Part model, mm, in its own coordinate system. Face numbers are marked on the shaded views. A direction names the side the tool comes from. Give positions to 0.01 mm unless a question says otherwise; leave off trailing zeros. Order: outer loops, then holes, each group sorted by start corner. A loop starts at its lowest first (then second) coordinate and runs counter-clockwise, first axis right, second up. Notation, with made-up numbers: (-5.5, -34.75) -> (8.5, -34.75) arc R30 ccw to (8.5, 3.25) -> close; hole circle Ø8 at (17, 66.25). An arc over 180 degrees is marked (long way). Write item = value, one per line. Start each with the question number.
(1) Saw through at A-A, the plane y = 0. List the corners of the cut face in (x, z), then the cut area to 3 significant figures.
(2) Which spindle directions (+Z, -Z, +X, -X, +Y, -Y) get a long thin tool onto all of the face, cutting with end or side? Do the marked faces 4 and 5. Say none if no direction does.
(3) Two-plate mould, pull along X, no slides. Class the marked faces 1, 2 and 3: pulls with the +X half, pulls with the -X half, needs draft (parallel to the pull), parting line crosses it, or undercut.
(4) Saw through at D-D, the plane z = -104. List the corners of the cut face in (x, y).
(5) Saw through at C-C, the plane z = -10. List the corners of the cut face in (x, y).
(6) Flat gauge pins, fed straight in: pin 1 (6 mm diameter, centred on x = 23.5, z = -104, fed in from -Y); pin 2 (12 mm diameter, centred on y = -24.5, z = -107, fed in from -X); pin 3 (8 mm diameter, centred on y = -6, z = -66.5, fed in from +X); pin 4 (12 mm diameter, centred on x = -2.5, y = 14, fed in from +Z). Where does each tip first touch, or does it go through?
(7) Probe line 1 along Y through (x, z) = (0, -35); line 2 along Y through (x, z) = (0, -107); line 3 along Z through (x, y) = (-27, 24). List the from-to ranges inside material, lowest first. Write a range as from..to.
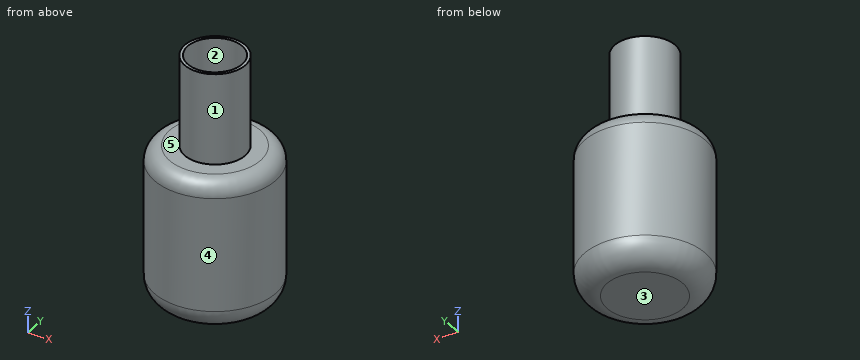
Autodesk Fusion 360 part; units mm, degrees
sketch "Sketch1" plane through (0, 0, 0) normal (0, 1, 0) x (1, 0, 0)
  line L0 (0, 0) -> (20, 0)
  line L1 (20, 0) -> (20, 60)
  line L2 (20, 60) -> (40, 60)
  line L3 (40, 60) -> (40, 160)
  line L4 (40, 160) -> (0, 160)
  line L5 (0, 160) -> (0, 0)
  dimension "d8" = 100
  dimension "d9" = 160
  dimension "d10" = 20
revolve "Revolve1" add sketch "Sketch1" angle 360 about axis through (0, 0, -160) along (0, 0, 1)
fillet "Fillet1" radius 10 1 edges at (-37.2931, -14.4646, -60)
fillet "Fillet2" radius 15 1 edges at (-37.2931, -14.4646, -160)
shell "Shell1" thickness 2 removed faces 1 at (3.8604, -3.2472, 0)
equation "overalheight = 160 mm"
equation "neckheight = 100 mm"
equation "fillet1 = 15 mm"
equation "fillet2 = 10 mm"
equation "fillet3 = 5 mm"
equation "diameter = 20 mm"
equation "wallthickness = 2 mm"
equation "d8 = neckheight"
equation "d9 = overalheight"
equation "d10 = diameter"
equation "d12 = fillet2"
equation "d13 = fillet1"
equation "d14 = wallthickness"
Results list:
q1.outline = (-40, -145) arc R15 ccw to (-25, -160) -> (25, -160) arc R15 ccw to (40, -145) -> (40, -70) arc R10 ccw to (30, -60) -> (20, -60) -> (20, 0) -> (18, 0) -> (18, -62) -> (30, -62) arc R8 cw to (38, -70) -> (38, -145) arc R13 cw to (25, -158) -> (-25, -158) arc R13 cw to (-38, -145) -> (-38, -70) arc R8 cw to (-30, -62) -> (-18, -62) -> (-18, 0) -> (-20, 0) -> (-20, -60) -> (-30, -60) arc R10 ccw to (-40, -70) -> close
q1.area = 833 mm^2
q2.face_4 = +Z, -Z
q2.face_5 = +Z
q3.face_1 = parting line crosses it
q3.face_2 = undercut
q3.face_3 = needs draft
q4.outline = circle Ø80 at (0, 0); hole circle Ø76 at (0, 0)
q5.outline = circle Ø40 at (0, 0); hole circle Ø36 at (0, 0)
q6.pin_1 = -34.35
q6.pin_2 = -35.46
q6.pin_3 = 39.85
q6.pin_4 = 0
q7.line_1 = -20..-18, 18..20
q7.line_2 = -40..-38, 38..40
q7.line_3 = -155.06..-151.73, -64.85..-62.1
